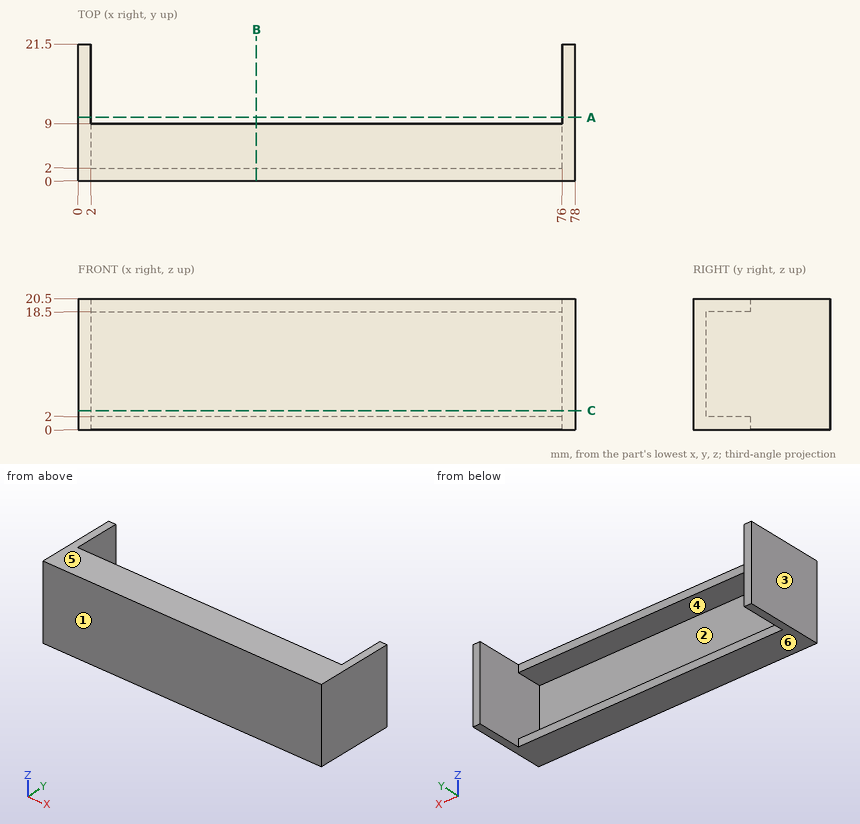
For this review, use the dimensioned drawing (mm, ordinates from the lowest corner) and the shaded views. A direction names the side the tool comes from. Give positions to 0.01 mm unless a question says otherwise; leave off trailing zeros. Write each loop counter-clockwise with the first axis right and the second up, starting at its lowest first coordinate (ties: lowest second). Pieces come first, ordered by that corner, then holes.
(1) Tool access review of the marked faces 1 and 2: name each direction out of +Z, -Z, +X, -X, +Y, -Y from which nothing blocks a thin tool from reaching the whole face with its end or side.
(2) For P1, Ø2, axis at x = 28, z = 0.5, coming from the +Y side; P2, Ø5, axis at x = 35.5, z = 12.5, coming from the +Y side, all flat-tipped, find the tip position at first contact; note any pin that passes through.
(3) Consider section B-B, the plane x = 28. Give the boundary of the cut face in (y, z), and give its area (3 significant figures).
(4) To check wall thickness, follow L1, parallel to X at y = 10.5, z = 19.5; L2, parallel to Z at x = 33, y = 6.25; L3, parallel to Y at x = 71.5, z = 4.25. State the ranges of each line that lie inside material, in increasing order.
(5) The part is to be moulded in two halves that separate along Z. For the marked faces 3, 4, 5 and 6, say which applies: released by +Z, released by -Z, zero draft, split by the parting line, or undercut.
(6) Consider section C-C, the plane z = 3. Give the boundary of the cut face in (x, y), and give its area (3 significant figures).
(7) Consider section A-A, the plane y = 10. Give the boundary of the cut face in (x, z).
Returned:
1. face 1: +Z, -Z, +X, -X, -Y
1. face 2: +Y
2. P1: stops at y = 9
2. P2: stops at y = 2
3. outline: (0, 0) - (9, 0) - (9, 2) - (2, 2) - (2, 18.5) - (9, 18.5) - (9, 20.5) - (0, 20.5) - close
3. area: 69.0 mm2
4. L1: x = 0 to 2, 76 to 78
4. L2: z = 0 to 2, 18.5 to 20.5
4. L3: y = 0 to 2
5. face 3: zero draft
5. face 4: undercut
5. face 5: released by +Z
5. face 6: released by -Z
6. outline: (0, 0) - (78, 0) - (78, 21.5) - (76, 21.5) - (76, 2) - (2, 2) - (2, 21.5) - (0, 21.5) - close
6. area: 234 mm2
7. outline: (0, 0) - (2, 0) - (2, 20.5) - (0, 20.5) - close; (76, 0) - (78, 0) - (78, 20.5) - (76, 20.5) - close
